from build123d import *

# Parameters (mm, degrees)
F0_W     = 32
F0_H     = 86.86
F1_DEPTH = 1.6
F2_R     = 3.1
F2_R_2   = 1.585
F2_W     = 5
F2_H     = 2.4618506432
F3_DEPTH = 25
F4_SIZE  = 1.27
F5_R     = 1.99999


# Not quite as in the source:
# - a fillet or chamfer is up to 0.001 mm smaller than in the source, because OpenCascade refuses the exact size


with BuildPart() as f1:
    # F0 (on Top) → F1 (new body)
    with BuildSketch(Plane.XY):
        Rectangle(F0_W, F0_H)
    extrude(amount=F1_DEPTH)

    # F2 (on face) → F3 (cut)
    with BuildSketch(Plane.XY.offset(1.6)):
        with Locations((-11.17, 35.05)):
            Circle(F2_R)
        with Locations((11.17, 35.05)):
            Circle(F2_R)
        with Locations((-11.17, -35.05)):
            Circle(F2_R)
        with Locations((11.17, -35.05)):
            Circle(F2_R)
        with BuildLine():
            Line((9.115, 28.49), (5.605, 28.49))
            ThreePointArc((5.605, 28.49), (5.0499211768, 28.2600788232), (4.82, 27.705))
            ThreePointArc((4.82, 27.705), (5.0499211768, 27.1499211768), (5.605, 26.92))
            Line((5.605, 26.92), (9.115, 26.92))
            ThreePointArc((9.115, 26.92), (9.6700788232, 27.1499211768), (9.9, 27.705))
            ThreePointArc((9.9, 27.705), (9.6700788232, 28.2600788232), (9.115, 28.49))
        make_face()
        with BuildLine():
            Line((-5.605, 28.49), (-9.115, 28.49))
            ThreePointArc((-9.115, 28.49), (-9.6700788232, 28.2600788232), (-9.9, 27.705))
            ThreePointArc((-9.9, 27.705), (-9.6700788232, 27.1499211768), (-9.115, 26.92))
            Line((-9.115, 26.92), (-5.605, 26.92))
            ThreePointArc((-5.605, 26.92), (-5.0499211768, 27.1499211768), (-4.82, 27.705))
            ThreePointArc((-4.82, 27.705), (-5.0499211768, 28.2600788232), (-5.605, 28.49))
        make_face()
        with Locations((16.825, 16.51)):
            Circle(F2_R_2)
        with Locations((16.825, 0)):
            Circle(F2_R_2)
        with Locations((16.825, -16.51)):
            Circle(F2_R_2)
        with Locations((-16.825, 0)):
            Circle(F2_R_2)
        with Locations((-16.825, 16.51)):
            Circle(F2_R_2)
        with Locations((-16.825, -16.51)):
            Circle(F2_R_2)
        with BuildLine():
            Line((-5.605, -26.92), (-9.115, -26.92))
            ThreePointArc((-9.115, -26.92), (-9.6700788232, -27.1499211768), (-9.9, -27.705))
            ThreePointArc((-9.9, -27.705), (-9.6700788232, -28.2600788232), (-9.115, -28.49))
            Line((-9.115, -28.49), (-5.605, -28.49))
            ThreePointArc((-5.605, -28.49), (-5.0499211768, -28.2600788232), (-4.82, -27.705))
            ThreePointArc((-4.82, -27.705), (-5.0499211768, -27.1499211768), (-5.605, -26.92))
        make_face()
        with BuildLine():
            Line((9.115, -26.92), (5.605, -26.92))
            ThreePointArc((5.605, -26.92), (5.0499211768, -27.1499211768), (4.82, -27.705))
            ThreePointArc((4.82, -27.705), (5.0499211768, -28.2600788232), (5.605, -28.49))
            Line((5.605, -28.49), (9.115, -28.49))
            ThreePointArc((9.115, -28.49), (9.6700788232, -28.2600788232), (9.9, -27.705))
            ThreePointArc((9.9, -27.705), (9.6700788232, -27.1499211768), (9.115, -26.92))
        make_face()
        with Locations((0, -42.6609253216)):
            Rectangle(F2_W, F2_H)
    extrude(amount=-F3_DEPTH, mode=Mode.SUBTRACT)

    # F4
    f4_edges = [f1.edges().sort_by_distance(p)[0] for p in [
        (16, 43.43, 0.8),
        (-16, 43.43, 0.8),
        (16, -43.43, 0.8),
        (-16, -43.43, 0.8),
    ]]
    chamfer(f4_edges, length=F4_SIZE)

    # F5 (radius 2 in the source; OpenCascade refuses exactly that, so slightly less here)
    f5_edges = [f1.edges().sort_by_distance(p)[0] for p in [
        (-2.5, -41.43, 0.8),
        (2.5, -41.43, 0.8),
    ]]
    fillet(f5_edges, radius=F5_R)


solid = f1.part
Work out the finished part from the listing and answer in its coordinate system (mm). A direction names the side the tool comes from. Coordinates: 2 decimals unless noted, no trailing zeros. Write each loop counter-clockwise with the first axis right and the second up, starting at its lowest first coordinate (ties: lowest second). Pieces come first, ordered by that corner, then holes. Notation, with made-up numbers: M -7.75,14 L 34.25,14 A16 cw 34.25,18 Z; hole C -40,-19.5 d5. An arc over 180 degrees is marked long. Use one line per item in the form item = value. Start each with the question number.
1. Straight lines are drawn through the part: probe 1 along Y at (x, z) = (11.17, 0.75); probe 2 along Y at (x, z) = (-8, 1.05); probe 3 along Y at (x, z) = (-8.5, 0.45). For each, find the intervals that lie inside material, in ascending order. Write a range as from..to.
2. The part is cut by section A-A (y = 35.05). Give the vertices of the cut face in (x, z).
3. A tool of negligible diameter and unlimited length cuts with its end or side. For faces 4 (the face through (-1.9, -42, 0.8)), 5 (the face through (-7, -28.49, 1)), 6 (the face through (16, 30, 1)), from which of +Z, -Z, +X, -X, +Y, -Y can it reach the whole face along a straight path? Write none if from no direction.
4. The mould has two halves that part along Y. Classify faces 1 (the face through (16, 8, 1)), 2 (the face through (9, -43.43, 1)), 3 (the face through (12.6, 32.3, 0.8)): released by +Y, released by -Y, zero draft, split by the parting line, or undercut.
5. The part is cut by section B-B (x = -11.17). Give the vertices of the cut face in (y, z), plus the area to 3 significant figures.
6. The part is cut by section C-C (z = 0.6). Give the number of separate pieces and of enclosed holes in the cut face, plus the area to 3 significant figures.
Evaluation:
q1.probe_1 = -43.43..-38.15, -31.95..31.95, 38.15..43.43
q1.probe_2 = -43.43..-28.49, -26.92..26.92, 28.49..43.43
q1.probe_3 = -43.43..-36.63, -33.47..-28.49, -26.92..26.92, 28.49..33.47, 36.63..43.43
q2.outline = M -16,0 L -14.27,0 L -14.27,1.6 L -16,1.6 Z; M -8.07,0 L 8.07,0 L 8.07,1.6 L -8.07,1.6 Z; M 14.27,0 L 16,0 L 16,1.6 L 14.27,1.6 Z
q3.face_4 = +Z, -Z, -Y
q3.face_5 = +Z, -Z
q3.face_6 = +Z, -Z, +X, +Y, -Y
q4.face_1 = zero draft
q4.face_2 = released by -Y
q4.face_3 = undercut
q5.outline = M -43.43,0 L -38.15,0 L -38.15,1.6 L -43.43,1.6 Z; M -31.95,0 L 31.95,0 L 31.95,1.6 L -31.95,1.6 Z; M 38.15,0 L 43.43,0 L 43.43,1.6 L 38.15,1.6 Z
q5.area = 119 mm^2
q6.separate_pieces = 1
q6.enclosed_holes = 8
q6.area = 2,610 mm^2
